Here's how the part is built. I have some questions about the finished solid (model axes, mm). Face numbers are marked on the shaded views. Give positions to 0.01 mm unless a question says otherwise; leave off trailing zeros. Write each loop counter-clockwise with the first axis right and the second up, starting at its lowest first coordinate (ties: lowest second). Pieces come first, ordered by that corner, then holes. Notation, with made-up numbers: (54, -38) -> (102, -38) arc R30 cw to (102, -15) -> close; hole circle Ø5 at (47.5, 82.5). An arc over 180 degrees is marked (long way). Use CSV: the item, a comma, the result in double quotes. Start each with the question number.
(1) If we mould it in two halves opening along X, with no side actions, what happens to the marked faces 1 and 2? For each: pulls with the +X half, pulls with the -X half, needs draft (parallel to the pull), parting line crosses it, or undercut.
(2) Suppose I cut it at A-A on y = -11.25. List the corners of the cut face in (x, z) for me.
(3) For pin 1 Ø2 at (x, y) = (-35, -13.5) entering from +Z; pin 2 Ø6 at (y, z) = (-5, 19) entering from -X; pin 3 Ø5 at (x, z) = (-37.5, 21) entering from +Y, each with a flat end and sliding along its axis, tell me the tip position at first contact or that it passes through.
(4) Suppose I cut it at D-D on z = -20. List the corners of the cut face in (x, y) for me.
(5) Suppose I cut it at B-B on x = -16.5. List the corners of the cut face in (y, z) for me.
(6) Suppose I cut it at C-C on x = -38.5. List the corners of the cut face in (y, z) for me, plus the area to 3 significant figures.
(7) I need wall thicknesses on L1, parallel to Y at x = -23.5, z = 17.5; L2, parallel to Z at x = -43, y = -6.75; L3, parallel to X at y = -12.25, z = -26.5. Which ranges of each line are inside material? Lowest first, please. Write a range as [from, to].
from build123d import *

# Parameters (mm, degrees)
F1_DEPTH = 15
F3_DEPTH = 13
F4_R     = 1.15
F5_DEPTH = 25


with BuildPart() as f1:
    # F0 (on Front) → F1 (new body)
    with BuildSketch(Plane.XZ):
        with BuildLine():
            ThreePointArc((-41.743332, -29.305931), (-40.329118, -28.720145), (-39.743332, -27.305931))
            ThreePointArc((-39.743332, -27.305931), (-40.156088, -26.089109), (-41.223989, -25.374537))
            ThreePointArc((-41.223989, -25.374537), (-43.726106, -27.044004), (-41.743332, -29.305931))
        make_face()
        with BuildLine():
            ThreePointArc((-41.223989, -25.374537), (-40.156088, -26.089109), (-39.743332, -27.305931))
            ThreePointArc((-39.743332, -27.305931), (-40.329118, -28.720145), (-41.743332, -29.305931))
            Line((-41.743332, -29.305931), (-13.743332, -29.305931))
            ThreePointArc((-13.743332, -29.305931), (-15.726106, -27.567859), (-14.262674, -25.374537))
            Line((-14.262674, -25.374537), (-27.743332, -25.374537))
            Line((-27.743332, -25.374537), (-31.169068, -25.374537))
            Line((-31.169068, -25.374537), (-41.223989, -25.374537))
        make_face()
        Polygon((-31.169068, 22.176644), (-31.169068, -25.374537), (-27.743332, -25.374537), (-21.045742, 21.713784), align=None)
        with BuildLine():
            ThreePointArc((-14.262674, -25.374537), (-15.726106, -27.567859), (-13.743332, -29.305931))
            ThreePointArc((-13.743332, -29.305931), (-12.329118, -28.720145), (-11.743332, -27.305931))
            ThreePointArc((-11.743332, -27.305931), (-12.526509, -25.718688), (-14.262674, -25.374537))
        make_face()
        with BuildLine():
            Line((-43.348153, 22.733499), (-31.169068, 22.176644))
            Line((-31.169068, 22.176644), (-21.045742, 21.713784))
            Line((-21.045742, 21.713784), (1.074161, 20.702413))
            ThreePointArc((1.074161, 20.702413), (-0.73886, 22.827734), (1.341411, 24.692272))
            Line((1.341411, 24.692272), (-43.06501, 26.575525))
            ThreePointArc((-43.06501, 26.575525), (-42.106774, 25.843711), (-41.743332, 24.694069))
            ThreePointArc((-41.743332, 24.694069), (-42.195695, 23.427253), (-43.348153, 22.733499))
        make_face()
        with BuildLine():
            ThreePointArc((-44.259922, 26.626201), (-45.690629, 24.237962), (-43.348153, 22.733499))
            ThreePointArc((-43.348153, 22.733499), (-42.195695, 23.427253), (-41.743332, 24.694069))
            ThreePointArc((-41.743332, 24.694069), (-42.106774, 25.843711), (-43.06501, 26.575525))
            Line((-43.06501, 26.575525), (-44.259922, 26.626201))
        make_face()
        with BuildLine():
            Line((1.256668, 20.694069), (1.074161, 20.702413))
            ThreePointArc((1.074161, 20.702413), (1.165319, 20.696156), (1.256668, 20.694069))
        make_face()
        with BuildLine():
            ThreePointArc((1.341411, 24.692272), (-0.73886, 22.827734), (1.074161, 20.702413))
            Line((1.074161, 20.702413), (1.256668, 20.694069))
            ThreePointArc((1.256668, 20.694069), (2.670882, 21.279855), (3.256668, 22.694069))
            ThreePointArc((3.256668, 22.694069), (2.700532, 24.077997), (1.341411, 24.692272))
        make_face()
        with BuildLine():
            ThreePointArc((-43.06501, 26.575525), (-43.658589, 26.692272), (-44.259922, 26.626201))
            Line((-44.259922, 26.626201), (-43.06501, 26.575525))
        make_face()
    extrude(amount=F1_DEPTH)

    # F2 (on face) → F3 (cut)
    with BuildSketch(Plane(origin=(0, 0, 0), x_dir=(-1, 0, 0), z_dir=(0, 1, 0))):
        with BuildLine():
            ThreePointArc((14.262674, -25.374537), (15.726106, -27.567859), (13.743332, -29.305931))
            Line((13.743332, -29.305931), (41.743332, -29.305931))
            ThreePointArc((41.743332, -29.305931), (39.760557, -27.567859), (41.223989, -25.374537))
            Line((41.223989, -25.374537), (31.169068, -25.374537))
            Line((31.169068, -25.374537), (31.169068, 22.176644))
            Line((31.169068, 22.176644), (43.348153, 22.733499))
            ThreePointArc((43.348153, 22.733499), (41.748741, 24.547075), (43.06501, 26.575525))
            Line((43.06501, 26.575525), (-1.341411, 24.692272))
            ThreePointArc((-1.341411, 24.692272), (0.73886, 22.827734), (-1.074161, 20.702413))
            Line((-1.074161, 20.702413), (21.045742, 21.713784))
            Line((21.045742, 21.713784), (27.743332, -25.374537))
            Line((27.743332, -25.374537), (14.262674, -25.374537))
        make_face()
    extrude(amount=-F3_DEPTH, mode=Mode.SUBTRACT)

    # F4 (on face) → F5 (cut)
    with BuildSketch(Plane.XZ.offset(15)):
        with Locations((-13.743332, -27.305931)):
            Circle(F4_R)
        with Locations((-41.743332, -27.305931)):
            Circle(F4_R)
        with Locations((1.256668, 22.694069)):
            Circle(F4_R)
        with Locations((-43.743332, 24.694069)):
            Circle(F4_R)
    extrude(amount=-F5_DEPTH, mode=Mode.SUBTRACT)


solid = f1.part
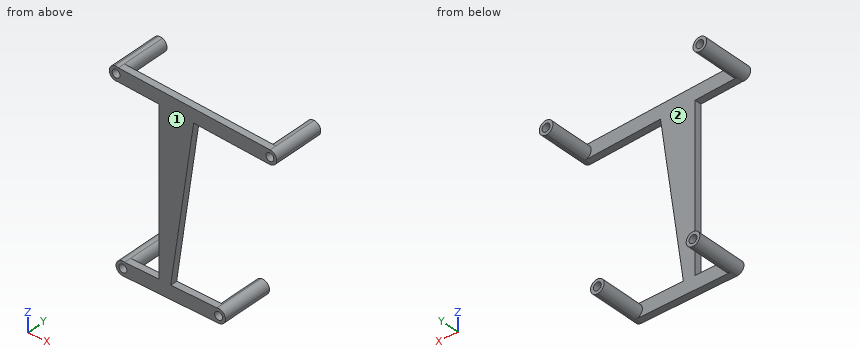
Geometry says:
1,face 1,"needs draft"
1,face 2,"undercut"
2,outline,"(-44.26, 26.63) arc R2 ccw (long way) to (-43.07, 26.58) arc R2 ccw to start; circle Ø4 at (-41.74, -27.31); (-13.74, -29.31) arc R2 ccw to (-11.74, -27.31) arc R2 ccw (long way) to start; (1.07, 20.7) arc R2 ccw to (1.26, 20.69) arc R2 ccw to (3.26, 22.69) arc R2 ccw to (1.34, 24.69) arc R2 ccw to start; hole circle Ø2.3 at (-43.74, 24.69); hole circle Ø2.3 at (-41.74, -27.31); hole circle Ø2.3 at (-13.74, -27.31); hole circle Ø2.3 at (1.26, 22.69)"
3,pin 1,"z = 26.28"
3,pin 2,"x = -0.62"
3,pin 3,"y = -13"
4,outline,"(-31.17, -15) -> (-26.98, -15) -> (-26.98, -13) -> (-31.17, -13) -> close"
5,outline,"(-15, -29.31) -> (-13, -29.31) -> (-13, -25.37) -> (-15, -25.37) -> close; (-15, 21.51) -> (-13, 21.51) -> (-13, 25.45) -> (-15, 25.45) -> close"
6,outline,"(-15, -29.31) -> (-13, -29.31) -> (-13, -25.37) -> (-15, -25.37) -> close; (-15, 22.51) -> (-13, 22.51) -> (-13, 26.38) -> (-15, 26.38) -> close"
6,area,"15.6 mm²"
7,L1,"[-15, -13]"
7,L2,"[-28.86, -25.75], [22.84, 23.82], [25.57, 26.55]"
7,L3,"[-43.57, -42.56], [-40.92, -39.91], [-15.57, -14.56], [-12.92, -11.91]"
